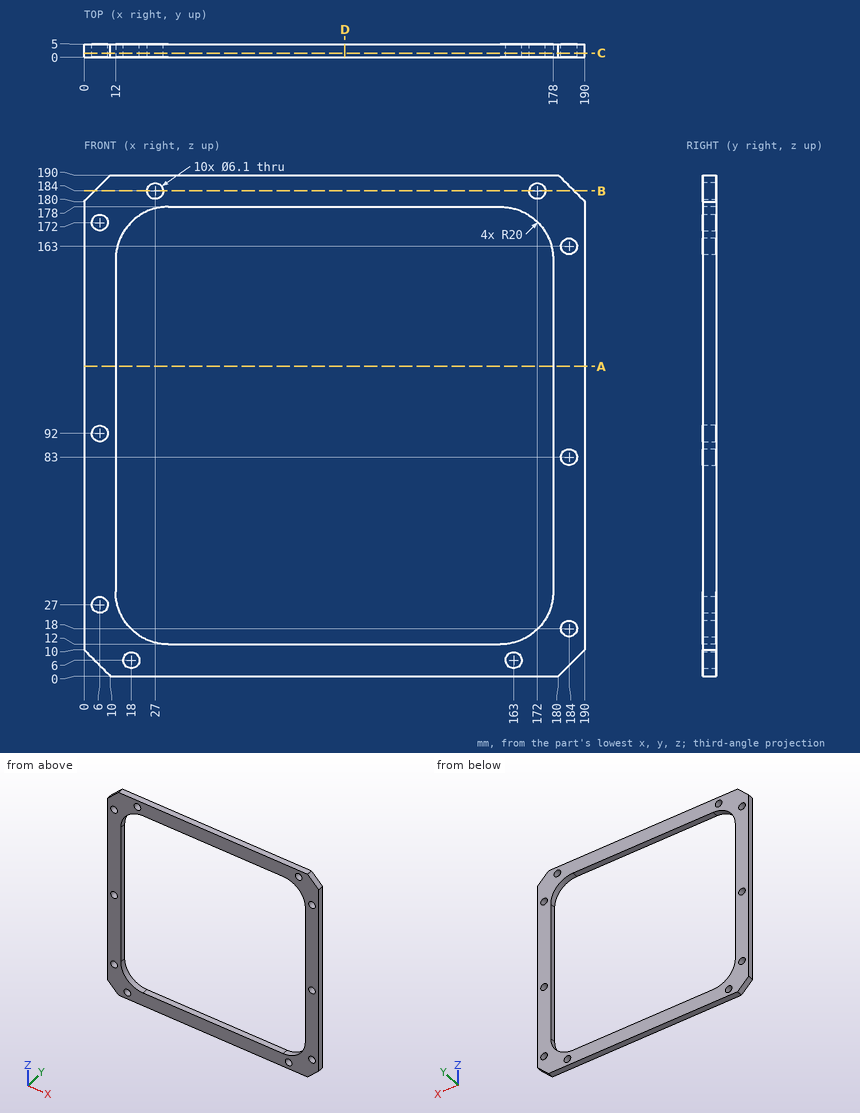
Study the drawing (mm; zero at the part's minimum x, y, z) and answer. Round coordinates to 2 decimals unless told otherwise and drop trailing zeros. Write each loop counter-clockwise with the first axis right and the second up, starting at its lowest first coordinate (ties: lowest second). Pieces come first, ordered by that corner, then holes.
1) A cutting plane is placed at B-B on z = 184. Determine the outline of the cut face in (x, y).
2) A cutting plane is placed at A-A on z = 117.5. Determine the outline of the cut face in (x, y), and give its area (3 significant figures).
3) Consider probe 1 along X at (y, z) = (2.75, 83); probe 2 along X at (y, z) = (3.65, 21.5); probe 3 along Z at (x, y) = (115, 1.35). Determine where each line is inside the solid, lowest interval first.
4) A cutting plane is placed at C-C on y = 1.55. Give the number of separate pieces and of enclosed holes in the cut face, and give its area (3 significant figures).
5) A cutting plane is placed at D-D on x = 99. Determine the outline of the cut face in (y, z), and give its area (3 significant figures).
Entries:
1. outline: (4, 0) - (23.95, 0) - (23.95, 5) - (4, 5) - close; (30.05, 0) - (168.95, 0) - (168.95, 5) - (30.05, 5) - close; (175.05, 0) - (186, 0) - (186, 5) - (175.05, 5) - close
2. outline: (0, 0) - (12, 0) - (12, 5) - (0, 5) - close; (178, 0) - (190, 0) - (190, 5) - (178, 5) - close
2. area: 120 mm2
3. probe 1: x = 0 to 12, 178 to 180.95, 187.05 to 190
3. probe 2: x = 0 to 14.98, 175.02 to 190
3. probe 3: z = 0 to 12, 178 to 190
4. separate pieces: 1
4. enclosed holes: 11
4. area: 8,400 mm2
5. outline: (0, 0) - (5, 0) - (5, 12) - (0, 12) - close; (0, 178) - (5, 178) - (5, 190) - (0, 190) - close
5. area: 120 mm2
